from build123d import *

# Parameters (mm, degrees)
SKETCH_1_W          = 32.5
SKETCH_1_H          = 46
EXTRUDE_1_DEPTH     = 14
SKETCH_2_W          = 10.2
SKETCH_2_H          = 6
CUT_EXTRUDE_2_DEPTH = 51.754925869
CUT_EXTRUDE_3_REACH = 33.449
SKETCH_4_R          = 1.65
SKETCH_5_R          = 1.25
CUT_EXTRUDE_4_DEPTH = 2
FILLET_1_R          = 2


with BuildPart() as part:
    # 草图1 → 凸台-拉伸1 (new body)
    with BuildSketch(Plane(origin=(0, 0, 0), x_dir=(1, 0, 0), z_dir=(0, 1, 0))):
        Rectangle(SKETCH_1_W, SKETCH_1_H)
    extrude(amount=EXTRUDE_1_DEPTH)

    # 草图2 → 切除-拉伸2 (cut, through all)
    with BuildSketch(Plane(origin=(0, 0, -23), x_dir=(-1, 0, 0), z_dir=(0, 0, -1))):
        with Locations((0, 11)):
            Rectangle(SKETCH_2_W, SKETCH_2_H)
        Polygon((5.1, 8), (-5.1, 8), (-10.6, 8), (-10.6, 3.4), (10.6, 3.4), (10.6, 8), align=None)
    extrude(amount=-CUT_EXTRUDE_2_DEPTH, mode=Mode.SUBTRACT)

    # 草图4 → 切除-拉伸3 (cut, up to next)
    with BuildSketch(Plane.XZ, mode=Mode.PRIVATE) as cut_extrude_3_sk1:
        with Locations(Location((-7.5, 5, 0), (0, 0, 270))):
            Circle(SKETCH_4_R)
    cut_extrude_3_tool1 = extrude(cut_extrude_3_sk1.sketch, amount=-CUT_EXTRUDE_3_REACH, mode=Mode.PRIVATE) & part.part
    # 草图4 → 切除-拉伸3 (cut, up to next)
    with BuildSketch(Plane.XZ, mode=Mode.PRIVATE) as cut_extrude_3_sk2:
        with Locations(Location((7.5, 5, 0), (0, 0, 270))):
            Circle(SKETCH_4_R)
    cut_extrude_3_tool2 = extrude(cut_extrude_3_sk2.sketch, amount=-CUT_EXTRUDE_3_REACH, mode=Mode.PRIVATE) & part.part
    # 草图4 → 切除-拉伸3 (cut, up to next)
    with BuildSketch(Plane.XZ, mode=Mode.PRIVATE) as cut_extrude_3_sk3:
        with Locations(Location((7.5, -5, 0), (0, 0, 270))):
            Circle(SKETCH_4_R)
    cut_extrude_3_tool3 = extrude(cut_extrude_3_sk3.sketch, amount=-CUT_EXTRUDE_3_REACH, mode=Mode.PRIVATE) & part.part
    # 草图4 → 切除-拉伸3 (cut, up to next)
    with BuildSketch(Plane.XZ, mode=Mode.PRIVATE) as cut_extrude_3_sk4:
        with Locations(Location((-7.5, -5, 0), (0, 0, 270))):
            Circle(SKETCH_4_R)
    cut_extrude_3_tool4 = extrude(cut_extrude_3_sk4.sketch, amount=-CUT_EXTRUDE_3_REACH, mode=Mode.PRIVATE) & part.part
    add(cut_extrude_3_tool1.solids().sort_by_distance((-7.5, 0, 5))[0], mode=Mode.SUBTRACT)
    add(cut_extrude_3_tool2.solids().sort_by_distance((7.5, 0, 5))[0], mode=Mode.SUBTRACT)
    add(cut_extrude_3_tool3.solids().sort_by_distance((7.5, 0, -5))[0], mode=Mode.SUBTRACT)
    add(cut_extrude_3_tool4.solids().sort_by_distance((-7.5, 0, -5))[0], mode=Mode.SUBTRACT)

    # 草图5 → 切除-拉伸4 (cut)
    with BuildSketch(Plane(origin=(0, 14, 0), x_dir=(1, 0, 0), z_dir=(0, 1, 0))):
        with Locations(Location((-10, 15, 0), (0, 0, 270))):
            Circle(SKETCH_5_R)
        with Locations(Location((10, 15, 0), (0, 0, 270))):
            Circle(SKETCH_5_R)
        with Locations(Location((10, -15, 0), (0, 0, 270))):
            Circle(SKETCH_5_R)
        with Locations(Location((-10, -15, 0), (0, 0, 270))):
            Circle(SKETCH_5_R)
    extrude(amount=-CUT_EXTRUDE_4_DEPTH, mode=Mode.SUBTRACT)

    # 圆角1
    fillet_1_edges = [part.edges().sort_by_distance(p)[0] for p in [
        (16.25, 0, 0),
        (-16.25, 0, 0),
    ]]
    fillet(fillet_1_edges, radius=FILLET_1_R)


solid = part.part
Part model, mm, in its own coordinate system. A direction names the side the tool comes from. Give positions to 0.01 mm unless a question says otherwise; leave off trailing zeros. Loops run counter-clockwise (first coordinate to the right, second up) from the corner with the lowest first, then second, coordinate; pieces in that order, holes last.
(1) Pull direction X, two halves, no side cores. Call faces 1 (the flat face through (0, 2, -23)), 2 (the cylindrical face through (-15.68, 0.6, -0.32)), 3 (the cylindrical face through (-8.5, 1.68, -3.69)), 4 (the flat face through (0, 3.4, 0)): pulls with the +X half, pulls with the -X half, needs draft (parallel to the pull), parting line crosses it, or undercut.
Return value:
face 1: needs draft
face 2: pulls with the -X half
face 3: undercut
face 4: undercut
(2) Pin check, flat tips, straight feed: pin 1 (2 mm diameter, centred on x = -7.5, z = -5, fed in from -Y); pin 2 (3 mm diameter, centred on x = -3.5, z = -11.5, fed in from +Y); pin 3 (1.5 mm diameter, centred on x = 10, z = -15, fed in from +Y). Stop position of each tip, or through.
Return value:
pin 1: stops at y = 8
pin 2: stops at y = 3.4
pin 3: stops at y = 12
(3) Band-saw the part on A-A (y = 7). Write the cut outline in (x, z).
Return value:
outline: (-16.25, -23) - (-10.6, -23) - (-10.6, 23) - (-16.25, 23) - close; (10.6, -23) - (16.25, -23) - (16.25, 23) - (10.6, 23) - close
(4) 3-axis set-ups, long thin cutter, end or side, ignore diameter. For faces 5 (the cylindrical face through (7.57, 1.68, -3.35)), 6 (the flat face through (-11, 14, 0)), 7 (the flat face through (10.6, 6, 0)), 8 (the cylindrical face through (11.24, 13.01, -15.16)): which of +Z, -Z, +X, -X, +Y, -Y reach the whole face in a straight line?
Return value:
face 5: -Y
face 6: +Z, -Z, +X, -X, +Y
face 7: +Z, -Z
face 8: +Y
(5) Drill centre lines: line 1 along X through (y, z) = (13.5, 15); line 2 along Y through (x, z) = (-7, 3); line 3 along X through (y, z) = (13, -7.5). Where is each one in solid material? Low to high.
Return value:
line 1: x = -16.25 to -11.25, -8.75 to -5.1, 5.1 to 8.75, 11.25 to 16.25
line 2: y = 0 to 3.4, 8 to 14
line 3: x = -16.25 to -5.1, 5.1 to 16.25
(6) Band-saw the part on D-D (z = 15). Write the cut outline in (x, y), and give its area (3 significant figures).
Return value:
outline: (-16.25, 2) arc R2 ccw to (-14.25, 0) - (14.25, 0) arc R2 ccw to (16.25, 2) - (16.25, 14) - (11.25, 14) - (11.25, 12) - (8.75, 12) - (8.75, 14) - (5.1, 14) - (5.1, 8) - (10.6, 8) - (10.6, 3.4) - (-10.6, 3.4) - (-10.6, 8) - (-5.1, 8) - (-5.1, 14) - (-8.75, 14) - (-8.75, 12) - (-11.25, 12) - (-11.25, 14) - (-16.25, 14) - close
area: 285 mm2
(7) Band-saw the part on B-B (x = 7.5). Write the cut outline in (y, z), and give its area (3 significant figures).
Return value:
outline: (0, -23) - (3.4, -23) - (3.4, -6.65) - (0, -6.65) - close; (0, -3.35) - (3.4, -3.35) - (3.4, 3.35) - (0, 3.35) - close; (0, 6.65) - (3.4, 6.65) - (3.4, 23) - (0, 23) - close; (8, -23) - (14, -23) - (14, 23) - (8, 23) - close
area: 410 mm2
(8) Band-saw the part on C-C (z = -5). Write the cut outline in (x, y).
Return value:
outline: (-16.25, 2) arc R2 ccw to (-14.25, 0) - (-9.15, 0) - (-9.15, 3.4) - (-10.6, 3.4) - (-10.6, 8) - (-5.1, 8) - (-5.1, 14) - (-16.25, 14) - close; (-5.85, 0) - (5.85, 0) - (5.85, 3.4) - (-5.85, 3.4) - close; (5.1, 8) - (10.6, 8) - (10.6, 3.4) - (9.15, 3.4) - (9.15, 0) - (14.25, 0) arc R2 ccw to (16.25, 2) - (16.25, 14) - (5.1, 14) - close
